Could you check a few things on this model? Use its own coordinates, in mm. A direction names the side the tool comes from. Coordinates: 2 decimals unless noted, no trailing zeros. Loops run counter-clockwise (first coordinate to the right, second up) from the corner with the lowest first, then second, coordinate; pieces in that order, holes last.
1) Imagine slicing it at A-A on y = 127. Please give me the cut outline in (x, z).
2) For faces 4 (the face through (1, 173.99, 3)), 5 (the face through (-11.381, 124.465, 4.472)), 6 (the face through (45.33, 131.77, 1.88)), which set-ups out of +Z, -Z, +X, -X, +Y, -Y let a thin tool reach every point of the face, with its end or its side?
3) If I drill on line 1 along Y through (x, z) = (-12.7, 4.8); line 2 along X through (y, z) = (135, 3.25); line 3 along Y through (x, z) = (-40, 3.25), over which ranges is the centre line in solid material (lowest first)?
4) Imagine slicing it at B-B on x = -12.7. Please give me the cut outline in (y, z).
5) Thinking about a two-plate mould opening in X: for faces 1 (the face through (-63.5, 86, 3)), 2 (the face through (-36.781, 48.265, 4.472)), 3 (the face through (1, 88, 0)), which applies, released by +X, released by -X, zero draft, split by the parting line, or undercut?
6) Will these pins go through, and if not, where does the flat tip stop? P1, Ø3, axis at x = -12, y = 127.5, coming from the +Z side; P2, Ø1.7, axis at x = 42.5, y = 132, coming from the -Z side.
```python
from build123d import *

# Parameters (mm, degrees)
BOSS_EXTRUDE1_DEPTH = 6.35
SKETCH3_R           = 2.8575
CUT_EXTRUDE1_DEPTH  = 3.81
SKETCH2_R           = 2.8575
CUT_EXTRUDE2_DEPTH  = 3.81


with BuildPart() as part:
    # Sketch1 → Boss-Extrude1 (new body)
    with BuildSketch(Plane.XY):
        Polygon((0, 173.99), (63.5, 173.99), (63.5, 0), (-63.5, 0), (-63.5, 173.99), align=None)
    extrude(amount=BOSS_EXTRUDE1_DEPTH)

    # Sketch3 → Cut-Extrude1 (cut)
    with BuildSketch(Plane.XY.offset(6.35)):
        with Locations((-38.1, 127)):
            Circle(SKETCH3_R)
        with Locations((-12.7, 127)):
            Circle(SKETCH3_R)
        with Locations((-38.1, 50.8)):
            Circle(SKETCH3_R)
        with Locations((-12.7, 50.8)):
            Circle(SKETCH3_R)
    extrude(amount=-CUT_EXTRUDE1_DEPTH, mode=Mode.SUBTRACT)

    # Sketch2 → Cut-Extrude2 (cut)
    with BuildSketch(Plane(origin=(0, 0, 0), x_dir=(-1, 0, 0), z_dir=(0, 0, -1))):
        with Locations((-43.064543118, 133.510265263)):
            Circle(SKETCH2_R)
        with Locations((-3.694543118, 133.510265263)):
            Circle(SKETCH2_R)
        with Locations((-43.064543118, 51.470265263)):
            Circle(SKETCH2_R)
        with Locations((-3.694543118, 51.470265263)):
            Circle(SKETCH2_R)
    extrude(amount=-CUT_EXTRUDE2_DEPTH, mode=Mode.SUBTRACT)


solid = part.part
```
Filled in:
1. outline: (-63.5, 0) - (63.5, 0) - (63.5, 6.35) - (-9.84, 6.35) - (-9.84, 2.54) - (-15.56, 2.54) - (-15.56, 6.35) - (-35.24, 6.35) - (-35.24, 2.54) - (-40.96, 2.54) - (-40.96, 6.35) - (-63.5, 6.35) - close
2. face 4: +Z, -Z, +X, -X, +Y
2. face 5: +Z
2. face 6: -Z
3. line 1: y = 0 to 47.94, 53.66 to 124.14, 129.86 to 173.99
3. line 2: x = -63.5 to 1.26, 6.13 to 40.63, 45.5 to 63.5
3. line 3: y = 0 to 48.67, 52.93 to 124.87, 129.13 to 173.99
4. outline: (0, 0) - (173.99, 0) - (173.99, 6.35) - (129.86, 6.35) - (129.86, 2.54) - (124.14, 2.54) - (124.14, 6.35) - (53.66, 6.35) - (53.66, 2.54) - (47.94, 2.54) - (47.94, 6.35) - (0, 6.35) - close
5. face 1: released by -X
5. face 2: undercut
5. face 3: zero draft
6. P1: stops at z = 2.54
6. P2: stops at z = 3.81
